Can you work these out from the model? Positions are in its coordinate system, mm. Face numbers are marked on the shaded views. A direction names the side the tool comes from. Round coordinates to 2 decimals unless told otherwise and drop trailing zeros. Loops run counter-clockwise (first coordinate to the right, second up) from the corner with the lowest first, then second, coordinate; pieces in that order, holes last.
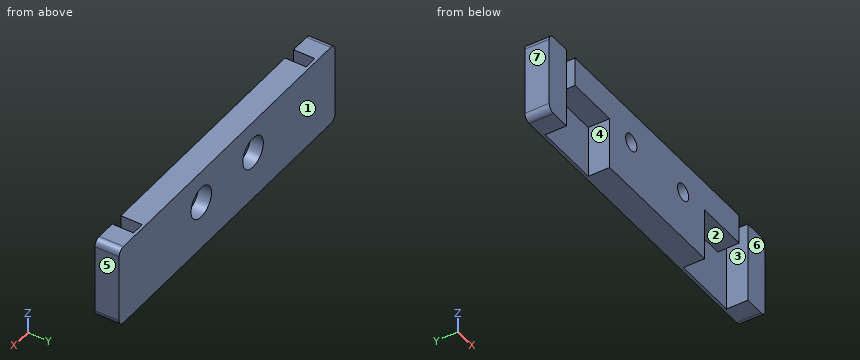
Autodesk Inventor part; units mm, degrees
ref_plane "YZ Plane" through (0, 0, 0) normal (1, 0, 0) x (0, 1, 0)
ref_plane "XZ Plane" through (0, 0, 0) normal (0, 1, 0) x (-1, 0, 0)
ref_plane "XY Plane" through (0, 0, 0) normal (0, 0, 1) x (1, 0, 0)
sketch "Sketch1" plane through (0, 0, 0) normal (0, 1, 0) x (-1, 0, 0)
  line L0 (50, -12.5) -> (-50, -12.5)
  line L1 (-50, -12.5) -> (-50, 12.5)
  line L2 (-50, 12.5) -> (50, 12.5)
  line L3 (50, 12.5) -> (50, -12.5)
  line L4 (50, -12.5) -> (-50, 12.5) construction
  line L5 (-50, -12.5) -> (50, 12.5) construction
  point P0 (0, 0)
  dimension "d0" = 100
  dimension "d1" = 25
extrude "Extrusion1" add sketch "Sketch1" along normal blind 7.4
sketch "Sketch2" plane through (0, 7.4, 0) normal (0, 1, 0) x (1, 0, 0)
  line L0 (-32.5, 12.8309) -> (-37.5, 12.8309)
  line L1 (-37.5, 12.8309) -> (-37.5, 27.8309)
  line L2 (-37.5, 27.8309) -> (-32.5, 27.8309)
  line L3 (-32.5, 27.8309) -> (-32.5, 12.8309)
  line L4 (32.5, 12.8309) -> (37.5, 12.8309)
  line L5 (32.5, 27.8309) -> (32.5, 12.8309)
  line L6 (37.5, 27.8309) -> (32.5, 27.8309)
  line L7 (37.5, 12.8309) -> (37.5, 27.8309)
  line L8 (-50, -12.5) -> (50, -12.5)
  line L9 (50, -12.5) -> (50, 12.5)
  line L10 (50, 12.5) -> (-50, 12.5)
  line L11 (-50, 12.5) -> (-50, -12.5)
  line L12 (-42, 12.5) -> (-22, 12.5)
  line L13 (-22, 12.5) -> (-22, -3.5)
  line L14 (-22, -3.5) -> (-42, -3.5)
  line L15 (-42, -3.5) -> (-42, 12.5)
  line L16 (-42, -3.5) -> (-42, -12.5)
  line L17 (-38, -3.5) -> (-38, -12.5)
  point P0 (0, 0)
  point P1 (-35, 12.8309)
  point P2 (-22, 12.5)
  dimension "d4" = 7
  dimension "d5" = 20
  dimension "d6" = 16
  dimension "d7" = 4
sketch "Sketch3" plane through (0, 7.4, 0) normal (0, 1, 0) x (1, 0, 0)
  line L0 (50, 12.5) -> (-50, 12.5)
  line L1 (-50, -12.5) -> (50, -12.5)
  line L2 (50, -12.5) -> (50, 12.5)
  line L3 (-50, 12.5) -> (-50, -12.5)
  point P0 (0, 0)
  point P1 (12, -2.5)
  dimension "d11" = 12
  dimension "d12" = 15
hole "Hole1" at (12, 7.4, 2.5) direction (0, -1, 0) diameter 5.2 end through all counterbore diameter 9.5 counterbore depth 4
fillet "Fillet1" radius 2 4 edges at (50, 3.7, 12.5) (50, 3.7, -12.5) (-50, 3.7, 12.5) (-50, 3.7, -12.5)
sketch "Sketch4" plane through (0, 0, 0) normal (0, -1, 0) x (1, 0, 0)
  line L0 (-22, -12.5) -> (-22, 3.5)
  line L1 (-22, 3.5) -> (-42, 3.5)
  line L2 (48, -12.5) -> (-48, -12.5)
  line L3 (-42, 3.5) -> (-42, -12.5)
  line L4 (-42, 3.5) -> (-42, 12.5)
  line L5 (-38, 3.5) -> (-38, 12.5)
  line L6 (-48, 12.5) -> (48, 12.5)
  point P0 (0, 0)
extrude "Extrusion3" cut sketch "Sketch4" against normal blind 6.5
mirror "Mirror2" about plane through (0, 0, 0) normal (1, 0, 0) of "Hole1", "Extrusion3"
properties part number "Limit Switch Bracket" material "ABS Plastic"
(1) If we section it at D-D, the plane y = 1.5: List the corners of the cut face in (x, z) for me.
Worked answers:
outline: (-50, -10.5) arc R2 ccw to (-48, -12.5) - (-42, -12.5) - (-42, 12.5) - (-48, 12.5) arc R2 ccw to (-50, 10.5) - close; (-38, 3.5) - (-22, 3.5) - (-22, -12.5) - (22, -12.5) - (22, 3.5) - (38, 3.5) - (38, 12.5) - (-38, 12.5) - close; (42, -12.5) - (48, -12.5) arc R2 ccw to (50, -10.5) - (50, 10.5) arc R2 ccw to (48, 12.5) - (42, 12.5) - close; hole circle Ø5.2 at (-12, 2.5); hole circle Ø5.2 at (12, 2.5)
(2) If we section it at A-A, the plane y = 5.25: List the corners of the cut face in (x, z) for me.
Worked answers:
outline: (-50, -10.5) arc R2 ccw to (-48, -12.5) - (-42, -12.5) - (-42, 12.5) - (-48, 12.5) arc R2 ccw to (-50, 10.5) - close; (-38, 3.5) - (-22, 3.5) - (-22, -12.5) - (22, -12.5) - (22, 3.5) - (38, 3.5) - (38, 12.5) - (-38, 12.5) - close; (42, -12.5) - (48, -12.5) arc R2 ccw to (50, -10.5) - (50, 10.5) arc R2 ccw to (48, 12.5) - (42, 12.5) - close; hole circle Ø9.5 at (-12, 2.5); hole circle Ø9.5 at (12, 2.5)
(3) If I drill on line 1 (X direction, y = 1.75, z = -1.75); line 2 (X direction, y = 5.85, z = 2.5); line 3 (X direction, y = 2.2, z = 2.5), over which ranges is the centre line in solid material (lowest first)?
Worked answers:
line 1: x = -50 to -42, -22 to 22, 42 to 50
line 2: x = -50 to -42, -22 to -16.75, -7.25 to 7.25, 16.75 to 22, 42 to 50
line 3: x = -50 to -42, -22 to -14.6, -9.4 to 9.4, 14.6 to 22, 42 to 50
(4) For the marked faces 1, 2 and 3, which set-ups out of +Z, -Z, +X, -X, +Y, -Y let a thin tool reach every point of the face, with its end or its side?
Worked answers:
face 1: +Z, -Z, +X, -X, +Y
face 2: -Z, -Y
face 3: +Z, -Z, -Y
(5) Will this pin go through, and if not, where does the flat tip stop? P1, Ø2, axis at x = -30, y = 3.5, coming from the -Z side.
Worked answers:
P1: stops at z = 3.5
(6) If we section it at C-C, the plane z = 2.5: List the corners of the cut face in (x, y) for me.
Worked answers:
outline: (-50, 0) - (-42, 0) - (-42, 6.5) - (-22, 6.5) - (-22, 0) - (-14.6, 0) - (-14.6, 3.4) - (-16.75, 3.4) - (-16.75, 7.4) - (-50, 7.4) - close; (-9.4, 0) - (9.4, 0) - (9.4, 3.4) - (7.25, 3.4) - (7.25, 7.4) - (-7.25, 7.4) - (-7.25, 3.4) - (-9.4, 3.4) - close; (14.6, 0) - (22, 0) - (22, 6.5) - (42, 6.5) - (42, 0) - (50, 0) - (50, 7.4) - (16.75, 7.4) - (16.75, 3.4) - (14.6, 3.4) - close
(7) If we mould it in two halves opening along X, with no side actions, what happens to the marked faces 4, 5, 6 and 7? For each: released by +X, released by -X, zero draft, split by the parting line, or undercut.
Worked answers:
face 4: undercut
face 5: released by +X
face 6: zero draft
face 7: released by -X
(8) If we section it at B-B, the plane x = -12: List the corners of the cut face in (y, z) for me, then the cut area to 3 significant figures.
Worked answers:
outline: (0, -12.5) - (7.4, -12.5) - (7.4, -2.25) - (3.4, -2.25) - (3.4, -0.1) - (0, -0.1) - close; (0, 5.1) - (3.4, 5.1) - (3.4, 7.25) - (7.4, 7.25) - (7.4, 12.5) - (0, 12.5) - close
area: 129 mm2
